Work out the finished part from the listing and answer in its coordinate system (mm). A direction names the side the tool comes from. Round coordinates to 2 decimals unless told otherwise and drop trailing zeros. Order: outer loops, then holes, each group sorted by start corner. A loop starts at its lowest first (then second) coordinate and runs counter-clockwise, first axis right, second up. Notation, with made-up numbers: (43, 33.5) - (88, 33.5) arc R20 ccw to (88, 58.5) - close; hole circle Ø4 at (82, 54). An arc over 180 degrees is marked (long way). One line per question, with ' | ' between items. Start each with the question number.
from build123d import *

# Parameters (mm, degrees)
F0_R     = 342.9
F1_DEPTH = 20.6375
F2_R     = 12.7
F3_DEPTH = 125.4125
F4_DEPTH = 38.1


with BuildPart() as f1:
    # F0 (on Right) → F1 (new body)
    with BuildSketch(Plane.YZ):
        Circle(F0_R)
    extrude(amount=-F1_DEPTH)

    # F2 (on face) → F3 (join)
    with BuildSketch(Plane(origin=(-20.6375, 0, 0), x_dir=(0, -1, 0), z_dir=(-1, 0, 0))):
        with Locations((249.618309, 46.975525)):
            Circle(F2_R)
        with Locations((-249.618309, 46.975525)):
            Circle(F2_R)
    extrude(amount=-F3_DEPTH)

    # F2 (on face) → F4 (join)
    with BuildSketch(Plane(origin=(-20.6375, 0, 0), x_dir=(0, -1, 0), z_dir=(-1, 0, 0))):
        with Locations((249.618309, 46.975525)):
            Circle(F2_R)
        with Locations((-249.618309, 46.975525)):
            Circle(F2_R)
    extrude(amount=F4_DEPTH)


solid = f1.part
1) Section C-C on x = -46 is taken. Give the vertices of the cut face in (y, z).
2) Flat-ended cylindrical pins translate along their axes: pin 1 (4 mm diameter, centred on y = 167, z = -85, fed in from -X); pin 2 (6 mm diameter, centred on x = -8, y = -234, fed in from -Z); pin 3 (6 mm diameter, centred on y = -241.5, z = -78.5, fed in from +X). Find the tip coordinate at first contact, or state that the pin passes through.
3) Section A-A on z = 0 is taken. Give the vertices of the cut face in (x, y), and give its area (3 significant figures).
4) For faces 1 (the cylindrical face through (-10.174, 184.341, 289.135)), 2 (the cylindrical face through (51.65, 259.7, 39.25)), 3 (the cylindrical face through (-39.42, 259.7, 39.25)), determine the directions among +Z, -Z, +X, -X, +Y, -Y from which every point of the face is accessible in a straight line to the end or side of a thin tool.
5) Straight lines are drawn through the part: line 1 (X direction, y = 29.5, z = 306); line 2 (Z direction, x = -20, y = -90.5); line 3 (Z direction, x = -4.5, y = -44). For each, find the intervals that lie inside material, in ascending order.
6) Section B-B on y = 254 is taken. Give the vertices of the cut face in (x, z) (1 decimal).
Recorded:
1) outline: circle Ø25.4 at (-249.62, 46.98); circle Ø25.4 at (249.62, 46.98)
2) pin 1: stops at x = -20.64 | pin 2: stops at z = -253.42 | pin 3: stops at x = 0
3) outline: (-20.64, -342.9) - (0, -342.9) - (0, 342.9) - (-20.64, 342.9) - close | area: 14,200 mm²
4) face 1: +X, -X | face 2: +X | face 3: -X
5) line 1: x = -20.64 to 0 | line 2: z = -330.74 to 330.74 | line 3: z = -340.07 to 340.07
6) outline: (-58.7, 35.1) - (-20.6, 35.1) - (-20.6, -230.4) - (0, -230.4) - (0, 35.1) - (104.8, 35.1) - (104.8, 58.9) - (0, 58.9) - (0, 230.4) - (-20.6, 230.4) - (-20.6, 58.9) - (-58.7, 58.9) - close
